Geometry check sheet. Reference: drawing and pictorial views, mm from the part's lowest x, y, z. Give positions to 0.01 mm unless a question says otherwise; leave off trailing zeros. Write each loop counter-clockwise with the first axis right and the second up, starting at its lowest first coordinate (ties: lowest second). Pieces come first, ordered by that corner, then holes. Notation, with made-up numbers: M -16,-17 L 39,-17 A31 ccw 39,17 Z; hole C 27,88.25 d7. An arc over 180 degrees is marked long. One line per item, written item: value. Start each with the question number.
1. Cross-section at C-C on x = 60. Record the cut outline in (y, z).
2. Scan lines: line 1 (Z direction, x = 42.5, y = 1.3); line 2 (Z direction, x = 42.5, y = 2.6); line 3 (Y direction, x = 36, z = 13). Record each from-to range of solid material in increasing order.
3. Cross-section at B-B on y = 3.5. Record the cut outline in (x, z), then the cut area to 3 significant figures.
4. Cross-section at A-A on x = 37.5. Record the cut outline in (y, z), then the cut area to 4 significant figures.
5. Gauge pin test, flat ends, axial feed: pin 1 (2 mm diameter, centred on y = 1, z = 24, fed in from +X); pin 2 (10 mm diameter, centred on x = 39.5, z = 34.5, fed in from -Y); pin 3 (2 mm diameter, centred on y = 1, z = 22.5, fed in from -X). Record the tip position at first contact, or that the pin passes through.
6. Cross-section at D-D on z = 42.5. Record the cut outline in (x, y).
7. Release check for a two-part mould opening along X. For the marked faces 1, 2 and 3 record: pulls with the +X half, pulls with the -X half, needs draft (parallel to the pull), parting line crosses it, or undercut.
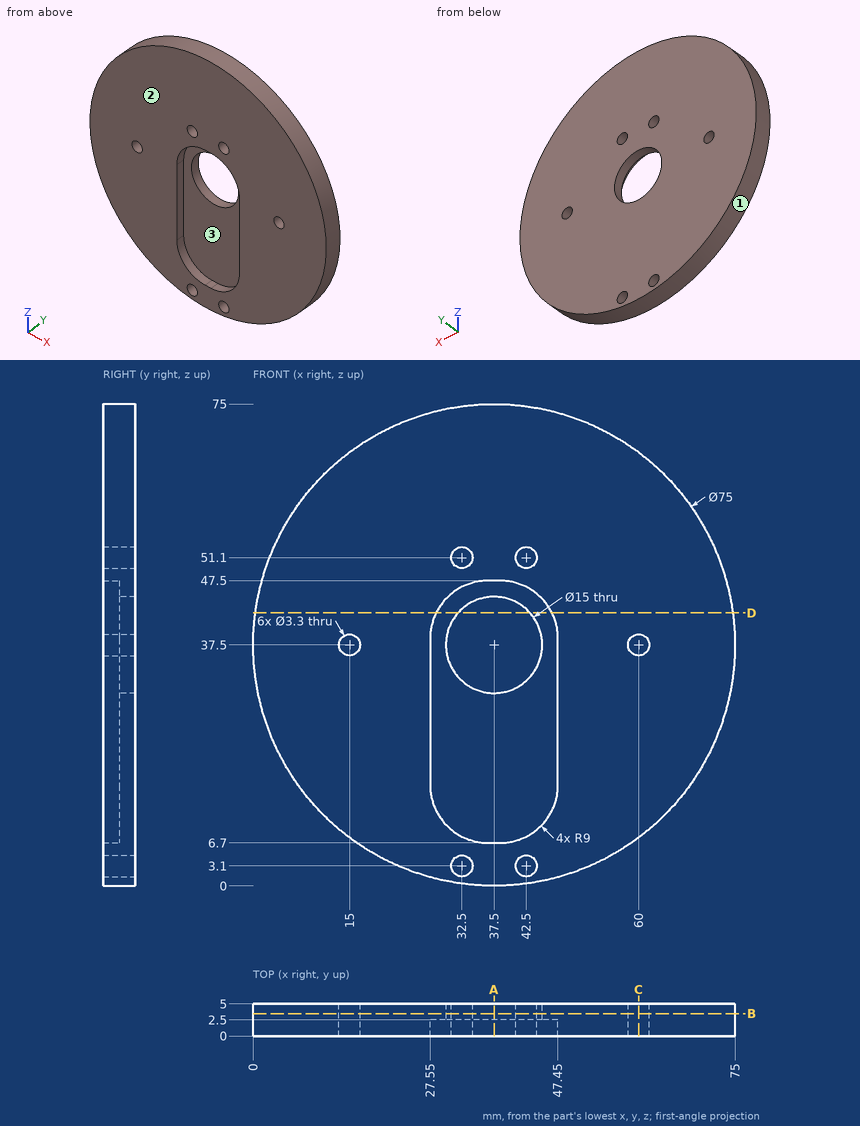
Report:
1. outline: M 0,7.5 L 5,7.5 L 5,35.85 L 0,35.85 Z; M 0,39.15 L 5,39.15 L 5,67.5 L 0,67.5 Z
2. line 1: z = 0.33 to 1.45, 4.75 to 7.66, 46.54 to 49.45, 52.75 to 74.67
2. line 2: z = 0.33 to 1.45, 4.75 to 31.91, 43.09 to 49.45, 52.75 to 74.67
2. line 3: y = 2.5 to 5
3. outline: C 37.5,37.5 d75; hole C 15,37.5 d3.3; hole C 37.5,37.5 d15; hole C 32.5,3.1 d3.3; hole C 32.5,51.1 d3.3; hole C 42.5,3.1 d3.3; hole C 42.5,51.1 d3.3; hole C 60,37.5 d3.3
3. area: 4,190 mm^2
4. outline: M 0,0 L 5,0 L 5,30 L 2.5,30 L 2.5,6.7 L 0,6.7 Z; M 0,47.5 L 2.5,47.5 L 2.5,45 L 5,45 L 5,75 L 0,75 Z
4. area: 235.5 mm^2
5. pin 1: stops at x = 72.86
5. pin 2: stops at y = 2.5
5. pin 3: stops at x = 2.71
6. outline: M 0.33,0 L 28.49,0 L 28.49,2.5 L 31.91,2.5 L 31.91,5 L 0.33,5 Z; M 43.09,2.5 L 46.51,2.5 L 46.51,0 L 74.67,0 L 74.67,5 L 43.09,5 Z
7. face 1: parting line crosses it
7. face 2: needs draft
7. face 3: undercut
